from build123d import *

# Parameters (mm, degrees)
F0_R     = 52.5
F0_R_2   = 17.5
F0_R_3   = 3.5
F1_DEPTH = 3
F4_R     = 2


with BuildPart() as f1:
    # F0 (on Top) → F1 (new body)
    with BuildSketch(Plane.XY):
        Circle(F0_R)
        with BuildLine():
            ThreePointArc((-22.4085, -32.543957), (-21.855421, -36.035962), (-25.347427, -36.589042))
            Line((-25.347427, -36.589042), (-26.965461, -35.413471))
            ThreePointArc((-26.965461, -35.413471), (-27.51854, -31.921465), (-24.026534, -31.368386))
            Line((-24.026534, -31.368386), (-22.4085, -32.543957))
        make_face(mode=Mode.SUBTRACT)
        with BuildLine():
            ThreePointArc((24.026534, -31.368386), (27.51854, -31.921465), (26.965461, -35.413471))
            Line((26.965461, -35.413471), (25.347427, -36.589042))
            ThreePointArc((25.347427, -36.589042), (21.855421, -36.035962), (22.4085, -32.543957))
            Line((22.4085, -32.543957), (24.026534, -31.368386))
        make_face(mode=Mode.SUBTRACT)
        with BuildLine():
            ThreePointArc((-37.875749, 11.255115), (-41.025933, 9.650016), (-42.631032, 12.8002))
            Line((-42.631032, 12.8002), (-42.012998, 14.702313))
            ThreePointArc((-42.012998, 14.702313), (-38.862814, 16.307412), (-37.257715, 13.157228))
            Line((-37.257715, 13.157228), (-37.875749, 11.255115))
        make_face(mode=Mode.SUBTRACT)
        Circle(F0_R_2, mode=Mode.SUBTRACT)
        with BuildLine():
            ThreePointArc((37.257715, 13.157228), (38.862814, 16.307412), (42.012998, 14.702313))
            Line((42.012998, 14.702313), (42.631032, 12.8002))
            ThreePointArc((42.631032, 12.8002), (41.025933, 9.650016), (37.875749, 11.255115))
            Line((37.875749, 11.255115), (37.257715, 13.157228))
        make_face(mode=Mode.SUBTRACT)
        with BuildLine():
            ThreePointArc((-1, 39.5), (-3.5, 42), (-1, 44.5))
            Line((-1, 44.5), (1, 44.5))
            ThreePointArc((1, 44.5), (3.5, 42), (1, 39.5))
            Line((1, 39.5), (-1, 39.5))
        make_face(mode=Mode.SUBTRACT)
        Circle(F0_R_2)
        Circle(F0_R_3, mode=Mode.SUBTRACT)
    extrude(amount=-F1_DEPTH)

    # F2 (on Front) → F3 (revolve)
    with BuildSketch(Plane.XZ):
        with BuildLine():
            Line((3.5, 5), (3.5, 0))
            Line((3.5, 0), (17.5, 0))
            add(Edge.make_bspline(
                [(3.5, 5), (12.593206, 5), (16.342813, 3.758031), (17.5, 0)],
                knots=[0, 0, 0, 0, 14.866069, 14.866069, 14.866069, 14.866069], degree=3))
        make_face()
    revolve(axis=Axis((0, 0, 2.5), (0, 0, -1)))

    # F4
    f4_edges = [f1.edges().sort_by_distance(p)[0] for p in [
        (-3.5, 0, 5),
    ]]
    fillet(f4_edges, radius=F4_R)


solid = f1.part
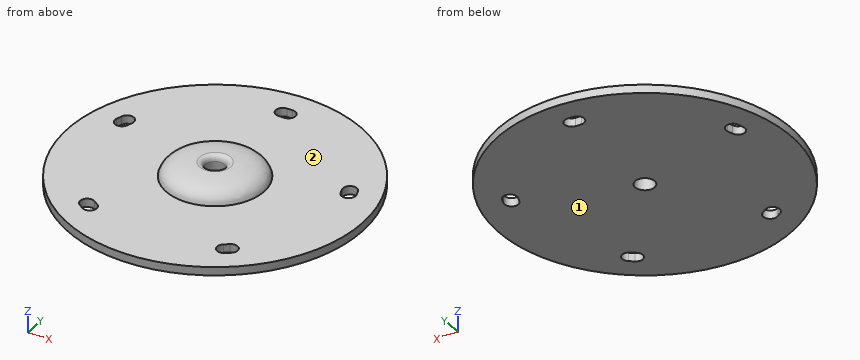
The model under review builds one solid part; all positions refer to its coordinate system, in mm. Face numbers are marked on the shaded views. A direction names the side the tool comes from. Coordinates: 2 decimals unless noted, no trailing zeros. Loops run counter-clockwise (first coordinate to the right, second up) from the corner with the lowest first, then second, coordinate; pieces in that order, holes last.
(1) Consider section A-A, the plane y = 42. Give the boundary of the cut face in (x, z).
Determined:
outline: (-31.5, -3) - (-3.5, -3) - (-3.5, 0) - (-31.5, 0) - close; (3.5, -3) - (31.5, -3) - (31.5, 0) - (3.5, 0) - close
(2) Tool access review of the marked faces 1 and 2: name each direction out of +Z, -Z, +X, -X, +Y, -Y from which nothing blocks a thin tool from reaching the whole face with its end or side.
Determined:
face 1: -Z, +X, -X, +Y, -Y
face 2: +Z
(3) Consider section D-D, the plane x = 46. Give the boundary of the cut face in (y, z).
Determined:
outline: (-25.3, -3) - (25.3, -3) - (25.3, 0) - (-25.3, 0) - close
(4) Consider section B-B, the plane z = -1.5. Give the boundary of the cut face in (x, y).
Determined:
outline: circle Ø105 at (0, 0); hole (-42.63, 12.8) arc R2.5 ccw to (-37.88, 11.26) - (-37.26, 13.16) arc R2.5 ccw to (-42.01, 14.7) - close; hole (-26.97, -35.41) - (-25.35, -36.59) arc R2.5 ccw to (-22.41, -32.54) - (-24.03, -31.37) arc R2.5 ccw to start; hole circle Ø7 at (0, 0); hole (-1, 39.5) - (1, 39.5) arc R2.5 ccw to (1, 44.5) - (-1, 44.5) arc R2.5 ccw to start; hole (22.41, -32.54) arc R2.5 ccw to (25.35, -36.59) - (26.97, -35.41) arc R2.5 ccw to (24.03, -31.37) - close; hole (37.26, 13.16) - (37.88, 11.26) arc R2.5 ccw to (42.63, 12.8) - (42.01, 14.7) arc R2.5 ccw to start
(5) Wall thickness on L1, parallel to Y at x = 0, z = -0.25; L2, parallel to Z at x = -48, y = -21; L3, parallel to X at y = 13, z = -1.5: over which ranges is each line inside the solid? List them lowest first.
Determined:
L1: y = -52.5 to -3.5, 3.5 to 39.5, 44.5 to 52.5
L2: z = -3 to 0
L3: x = -50.87 to -42.57, -37.31 to 37.31, 42.57 to 50.87
(6) Insertion check: P1, Ø2, axis at x = 0.5, z = -1.5, coming from the -Y side; P2, Ø1.6, axis at x = -0.5, z = -2, coming from the +Y side; P3, Ø1, axis at x = 31.5, y = 10.5, coming from the +Z side. Each pin has a flat end and moves straight along its axis. Give the tip position at first contact, or say it passes through.
Determined:
P1: stops at y = -52.5
P2: stops at y = 52.5
P3: stops at z = 0
(7) Consider section C-C, the plane x = 19. Give the boundary of the cut face in (y, z), plus the area to 3 significant figures.
Determined:
outline: (-48.94, -3) - (48.94, -3) - (48.94, 0) - (-48.94, 0) - close
area: 294 mm2
